Read the model definition and answer for the solid it produces. Units are mm, in the model's axes. Face numbers are marked on the shaded views. Coordinates: 2 decimals unless noted, no trailing zeros. Write each loop counter-clockwise with the first axis right and the second up, starting at its lowest first coordinate (ties: lowest second). Pieces come first, ordered by that corner, then holes. Notation, with made-up numbers: (38, 18) -> (92, 18) arc R23 cw to (92, 54) -> close; hole circle Ø3 at (71.25, -23). An arc over 180 degrees is marked (long way). Answer in a Markdown table with one row per item. Add a question column.
Item 1: Straight lines are drawn through the part: line 1 (Z direction, x = 0, y = 6.5); line 2 (X direction, y = 35, z = -0.5); line 3 (Z direction, x = 24, y = 96). For each, find the intervals that lie inside material, in ascending order. Write a range as from..to.
Item 2: Section A-A on x = 0 is taken. Write down the section's boundary in (y, z), then the cut area to 3 significant figures.
Item 3: Given pin 1 Ø2 at (y, z) = (86.5, -15.5) entering from -X; pin 2 Ø12 at (x, y) = (-22.5, 11) entering from +Z; pin 3 Ø8 at (y, z) = (37, 24.5) entering from +X, each flat-ended and moving along its own axis, determine where each tip first touches the part or whether it passes through.
Item 4: For a pull along Z with two mould halves and no side action, classify the marked faces 1 and 2 as +Z half, -Z half, draft (parallel to the pull), parting line (faces both ways), or undercut.
Item 5: Section B-B on y = 19 is taken. Write down the section's boundary in (x, z), then the cut area to 3 significant figures.
```python
from build123d import *

# Parameters (mm, degrees)
F0_R     = 37
F1_DEPTH = 100
F2_R     = 34
F3_DEPTH = 245
F4_R     = 2
F5_R     = 35.5
F6_DEPTH = 10


with BuildPart() as f1:
    # F0 (on Front) → F1 (new body)
    with BuildSketch(Plane.XZ):
        Circle(F0_R)
    extrude(amount=-F1_DEPTH)

    # F2 (on face) → F3 (cut)
    with BuildSketch(Plane.XZ):
        Circle(F2_R)
    extrude(amount=-F3_DEPTH, mode=Mode.SUBTRACT)

    # F4
    f4_edges = [f1.edges().sort_by_distance(p)[0] for p in [
        (-37, 100, 0),
    ]]
    fillet(f4_edges, radius=F4_R)

    # F5 (on Front) → F6 (cut)
    with BuildSketch(Plane.XZ):
        Circle(F5_R)
    extrude(amount=-F6_DEPTH, mode=Mode.SUBTRACT)


solid = f1.part
```
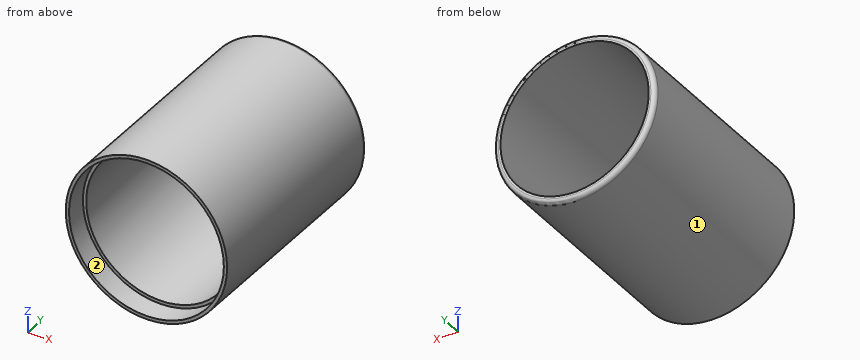
Results below:
| question | item | result |
|---|---|---|
| 1 | line 1 | z = -37..-35.5, 35.5..37 |
| 1 | line 2 | x = -37..-34, 34..37 |
| 1 | line 3 | z = -28.16..-24.08, 24.08..28.16 |
| 2 | outline | (0, -37) -> (98, -37) arc R2 ccw to (100, -35) -> (100, -34) -> (10, -34) -> (10, -35.5) -> (0, -35.5) -> close; (0, 35.5) -> (10, 35.5) -> (10, 34) -> (100, 34) -> (100, 35) arc R2 ccw to (98, 37) -> (0, 37) -> close |
| 2 | area | 568 mm2 |
| 3 | pin 1 | stops at x = -34.04 |
| 3 | pin 2 | stops at z = 33.12 |
| 3 | pin 3 | stops at x = 30.8 |
| 4 | face 1 | parting line |
| 4 | face 2 | undercut |
| 5 | outline | circle Ø74 at (0, 0); hole circle Ø68 at (0, 0) |
| 5 | area | 669 mm2 |
